from build123d import *

# Parameters (mm, degrees)
SKETCH_1_R      = 1.55
SKETCH_1_W      = 118
SKETCH_1_H      = 2.75
SKETCH_1_W_2    = 2.75
SKETCH_1_H_2    = 118
EXTRUDE_2_DEPTH = 3


with BuildPart() as part:
    # 草图1 → 凸台-拉伸2 (new body)
    with BuildSketch(Plane.XY):
        with BuildLine():
            Line((208.75, -2.75), (208.75, 202.75))
            ThreePointArc((208.75, 202.75), (206.992640687, 206.992640687), (202.75, 208.75))
            Line((202.75, 208.75), (-2.75, 208.75))
            ThreePointArc((-2.75, 208.75), (-6.992640687, 206.992640687), (-8.75, 202.75))
            Line((-8.75, 202.75), (-8.75, -2.75))
            ThreePointArc((-8.75, -2.75), (-6.992640687, -6.992640687), (-2.75, -8.75))
            Line((-2.75, -8.75), (202.75, -8.75))
            ThreePointArc((202.75, -8.75), (206.992640687, -6.992640687), (208.75, -2.75))
        make_face()
        with Locations((5, 195)):
            Circle(SKETCH_1_R, mode=Mode.SUBTRACT)
        with Locations((195, 195)):
            Circle(SKETCH_1_R, mode=Mode.SUBTRACT)
        with Locations((195, 5)):
            Circle(SKETCH_1_R, mode=Mode.SUBTRACT)
        with Locations((5, 5)):
            Circle(SKETCH_1_R, mode=Mode.SUBTRACT)
        with Locations((95, 100)):
            Circle(SKETCH_1_R, mode=Mode.SUBTRACT)
        with Locations((105, 100)):
            Circle(SKETCH_1_R, mode=Mode.SUBTRACT)
        with Locations((39, 12)):
            Circle(SKETCH_1_R, mode=Mode.SUBTRACT)
        with Locations((61, 12)):
            Circle(SKETCH_1_R, mode=Mode.SUBTRACT)
        with Locations((139, 12)):
            Circle(SKETCH_1_R, mode=Mode.SUBTRACT)
        with Locations((161, 12)):
            Circle(SKETCH_1_R, mode=Mode.SUBTRACT)
        with Locations((188, 39)):
            Circle(SKETCH_1_R, mode=Mode.SUBTRACT)
        with Locations((188, 61)):
            Circle(SKETCH_1_R, mode=Mode.SUBTRACT)
        with Locations((188, 161)):
            Circle(SKETCH_1_R, mode=Mode.SUBTRACT)
        with Locations((188, 139)):
            Circle(SKETCH_1_R, mode=Mode.SUBTRACT)
        with Locations((39, 188)):
            Circle(SKETCH_1_R, mode=Mode.SUBTRACT)
        with Locations((61, 188)):
            Circle(SKETCH_1_R, mode=Mode.SUBTRACT)
        with Locations((139, 188)):
            Circle(SKETCH_1_R, mode=Mode.SUBTRACT)
        with Locations((161, 188)):
            Circle(SKETCH_1_R, mode=Mode.SUBTRACT)
        with Locations((12, 161)):
            Circle(SKETCH_1_R, mode=Mode.SUBTRACT)
        with Locations((12, 139)):
            Circle(SKETCH_1_R, mode=Mode.SUBTRACT)
        with Locations((12, 61)):
            Circle(SKETCH_1_R, mode=Mode.SUBTRACT)
        with Locations((12, 39)):
            Circle(SKETCH_1_R, mode=Mode.SUBTRACT)
        Polygon((0, 202.75), (0, 205.75), (20, 205.75), (20, 202.75), (10, 202.75), (10, 200), (4, 200), (4, 202.75), align=None, mode=Mode.SUBTRACT)
        Polygon((4, 0), (10, 0), (10, -2.75), (20, -2.75), (20, -5.75), (0, -5.75), (0, -2.75), (4, -2.75), align=None, mode=Mode.SUBTRACT)
        Polygon((0, 4), (0, 10), (-2.75, 10), (-2.75, 20), (-5.75, 20), (-5.75, 0), (-2.75, 0), (-2.75, 4), align=None, mode=Mode.SUBTRACT)
        Polygon((200, 4), (200, 10), (202.75, 10), (202.75, 20), (205.75, 20), (205.75, 0), (202.75, 0), (202.75, 4), align=None, mode=Mode.SUBTRACT)
        Polygon((200, 202.75), (200, 205.75), (180, 205.75), (180, 202.75), (190, 202.75), (190, 200), (196, 200), (196, 202.75), align=None, mode=Mode.SUBTRACT)
        Polygon((202.75, 200), (205.75, 200), (205.75, 180), (202.75, 180), (202.75, 190), (200, 190), (200, 196), (202.75, 196), align=None, mode=Mode.SUBTRACT)
        Polygon((200, -2.75), (200, -5.75), (180, -5.75), (180, -2.75), (190, -2.75), (190, 0), (196, 0), (196, -2.75), align=None, mode=Mode.SUBTRACT)
        with Locations((100, -1.375)):
            Rectangle(SKETCH_1_W, SKETCH_1_H, mode=Mode.SUBTRACT)
        with Locations((201.375, 100)):
            Rectangle(SKETCH_1_W_2, SKETCH_1_H_2, mode=Mode.SUBTRACT)
        with Locations((100, 201.375)):
            Rectangle(SKETCH_1_W, SKETCH_1_H, mode=Mode.SUBTRACT)
        Polygon((-2.75, 200), (-5.75, 200), (-5.75, 180), (-2.75, 180), (-2.75, 190), (0, 190), (0, 196), (-2.75, 196), align=None, mode=Mode.SUBTRACT)
        with Locations((-1.375, 100)):
            Rectangle(SKETCH_1_W_2, SKETCH_1_H_2, mode=Mode.SUBTRACT)
    extrude(amount=EXTRUDE_2_DEPTH)


solid = part.part
CAD build for the part. Positions are in the model's coordinates, mm. Round coordinates to 2 decimals unless told otherwise and drop trailing zeros. Write each loop counter-clockwise with the first axis right and the second up, starting at its lowest first coordinate (ties: lowest second). Pieces come first, ordered by that corner, then holes.
(1) Drop flat-ended pins along their axis: P1, Ø2.5, axis at x = 139, y = 188, coming from the -Z side; P2, Ø5, axis at x = 195, y = 195, coming from the -Z side; P3, Ø1.5, axis at y = 204, z = 1, coming from the +X side. Give the stop position or say it passes through.
(2) Slice it at A-A, the plane y = 133.5. Write the cut outline in (x, z), and give its area (3 significant figures).
(3) Slice it at B-B, the plane z = 1.8. Count the separate pieces of the cut face and the enclosed holes in it, and give its area (3 significant figures).
(4) Probe line 1 along Y through (x, z) = (72, 0.75); line 2 along X through (y, z) = (192, 2.85). List the from-to ranges inside material, lowest first.
From the geometry:
1. P1: passes through
1. P2: stops at z = 0
1. P3: stops at x = 208.73
2. outline: (-8.75, 0) - (-2.75, 0) - (-2.75, 3) - (-8.75, 3) - close; (0, 0) - (200, 0) - (200, 3) - (0, 3) - close; (202.75, 0) - (208.75, 0) - (208.75, 3) - (202.75, 3) - close
2. area: 636 mm2
3. separate pieces: 1
3. enclosed holes: 34
3. area: 45,200 mm2
4. line 1: y = -8.75 to -2.75, 0 to 200, 202.75 to 208.75
4. line 2: x = -8.75 to -5.75, 0 to 200, 205.75 to 208.75
